Geometry check sheet. Reference: the model listing, model coordinates, mm. A direction names the side the tool comes from. Round coordinates to 2 decimals unless told otherwise and drop trailing zeros. Write each loop counter-clockwise with the first axis right and the second up, starting at its lowest first coordinate (ties: lowest second). Pieces come first, ordered by that corner, then holes. Notation, with made-up numbers: (-25, -6) -> (-5, -6) arc R16 cw to (-5, 20) -> close; hole circle Ø10 at (-35.5, 64.25). An arc over 180 degrees is marked (long way). Return JSON: item names as keys, results as strings. Group by question number.
from build123d import *

# Parameters (mm, degrees)
SKETCH1_W           = 22.2
SKETCH1_H           = 11.8
BOSS_EXTRUDE1_DEPTH = 22
SKETCH2_W           = 5
SKETCH2_H           = 2
BOSS_EXTRUDE2_DEPTH = 11.8
BOSS_EXTRUDE3_DEPTH = 4
SKETCH5_R           = 3.5
BOSS_EXTRUDE5_DEPTH = 2
SKETCH6_R           = 0.75
CUT_EXTRUDE2_DEPTH  = 2


with BuildPart() as part:
    # Sketch1 → Boss-Extrude1 (new body)
    with BuildSketch(Plane(origin=(0, 0, 0), x_dir=(1, 0, 0), z_dir=(0, 1, 0))):
        Rectangle(SKETCH1_W, SKETCH1_H)
    extrude(amount=-BOSS_EXTRUDE1_DEPTH)

    # Sketch2 → Boss-Extrude2 (add)
    with BuildSketch(Plane.XY.offset(5.9)):
        with Locations((13.6, -5)):
            Rectangle(SKETCH2_W, SKETCH2_H)
        with Locations((-13.6, -5)):
            Rectangle(SKETCH2_W, SKETCH2_H)
    extrude(amount=-BOSS_EXTRUDE2_DEPTH)

    # Sketch4 → Boss-Extrude3 (add)
    with BuildSketch(Plane(origin=(0, 0, 0), x_dir=(1, 0, 0), z_dir=(0, 1, 0))):
        with BuildLine():
            ThreePointArc((0.119, -2.998906301), (11.1, 0), (0.119, 2.998906301))
            ThreePointArc((0.119, 2.998906301), (-2.8, 0), (0.119, -2.998906301))
        make_face()
    extrude(amount=BOSS_EXTRUDE3_DEPTH)

    # Sketch5 → Boss-Extrude5 (add)
    with BuildSketch(Plane(origin=(0, 4, 0), x_dir=(1, 0, 0), z_dir=(0, 1, 0))):
        with Locations(Location((5.2, 0, 0), (0, 0, 270))):
            Circle(SKETCH5_R)
    extrude(amount=BOSS_EXTRUDE5_DEPTH)

    # Sketch6 → Cut-Extrude2 (cut)
    with BuildSketch(Plane(origin=(0, -4, 0), x_dir=(1, 0, 0), z_dir=(0, 1, 0))):
        with Locations(Location((-13.6, 0, 0), (0, 0, 270))):
            Circle(SKETCH6_R)
        with Locations(Location((13.6, 0, 0), (0, 0, 270))):
            Circle(SKETCH6_R)
    extrude(amount=-CUT_EXTRUDE2_DEPTH, mode=Mode.SUBTRACT)


solid = part.part
1) Mould release check, pull along X, two halves, no side actions. Record for faces 1 (the face through (-15, -4, 0)), 2 (the face through (11.1, -2, 0)), 3 (the face through (-11.1, -14, 0)), 4 (the face through (-12.968, -4.986, 0.403)): +X half, -X half, draft (parallel to the pull), parting line (faces both ways), or undercut.
2) Sectioned sample at A-A on x = -13.6. Enter the section's corners in (y, z), and give its area (3 significant figures).
3) Sectioned sample at C-C on x = 3. Enter the section's corners in (y, z).
4) Go/stop test with flat-tipped pins: P1, Ø2, axis at y = -2, z = 0, coming from the +X side; P2, Ø6, axis at y = -16, z = -2.5, coming from the -X side; P3, Ø1.7, axis at x = 13.6, z = 0, coming from the +Y side; P4, Ø0.9, axis at x = -13.6, z = 0, coming from the -Y side. Record where each tip stops, or that it passes through.
5) Tool access check on faces 5 (the face through (10, 0, 5)), 6 (the face through (11.1, -14, 0)), 7 (the face through (1.783, 4.986, -0.759)), 8 (the face through (-11.1, -2, 0)). Record the directions out of +Z, -Z, +X, -X, +Y, -Y that give a thin tool (end or side, any length) a straight path to the whole face; none if there is none.
6) Sectioned sample at D-D on y = -10.25. Enter the section's corners in (x, z).
7) Material ranges on probe 1 along X at (y, z) = (-4.95, 0); probe 2 along X at (y, z) = (-19.75, -2.25); probe 3 along Y at (x, z) = (5.5, -5), recorded low to high. Write a range as [from, to].
8) Sectioned sample at B-B on z = -4. Enter the section's corners in (x, y), and give its area (3 significant figures).
Evaluation:
{
 "1": {"face 1": "draft", "face 2": "+X half", "face 3": "-X half", "face 4": "undercut"},
 "2": {"outline": "(-6, -5.9) -> (-4, -5.9) -> (-4, -0.75) -> (-6, -0.75) -> close; (-6, 0.75) -> (-4, 0.75) -> (-4, 5.9) -> (-6, 5.9) -> close", "area": "20.6 mm2"},
 "3": {"outline": "(-22, -5.9) -> (0, -5.9) -> (0, -5.47) -> (4, -5.47) -> (4, -2.72) -> (6, -2.72) -> (6, 2.72) -> (4, 2.72) -> (4, 5.47) -> (0, 5.47) -> (0, 5.9) -> (-22, 5.9) -> close"},
 "4": {"P1": "stops at x = 11.1", "P2": "stops at x = -11.1", "P3": "stops at y = -4", "P4": "passes through"},
 "5": {"face 5": "+Z, +X, +Y", "face 6": "+Z, -Z, +X, -Y", "face 7": "+Y", "face 8": "+Z, -Z, -X, +Y"},
 "6": {"outline": "(-11.1, -5.9) -> (11.1, -5.9) -> (11.1, 5.9) -> (-11.1, 5.9) -> close"},
 "7": {"probe 1": "x = [-16.1, -14.35], [-12.85, 12.85], [14.35, 16.1]", "probe 2": "x = [-11.1, 11.1]", "probe 3": "y = [-22, 4]"},
 "8": {"outline": "(-16.1, -6) -> (-11.1, -6) -> (-11.1, -22) -> (11.1, -22) -> (11.1, -6) -> (16.1, -6) -> (16.1, -4) -> (11.1, -4) -> (11.1, 0) -> (9.54, 0) -> (9.54, 4) -> (0.86, 4) -> (0.86, 0) -> (-11.1, 0) -> (-11.1, -4) -> (-16.1, -4) -> close", "area": "543 mm2"}
}
